from build123d import *

# Parameters (mm, degrees)
F0_W        = 5
F0_H        = 62.5
F0_H_2      = 5
F0_W_2      = 60
F1_DEPTH    = 10.5
F2_W        = 5
F2_H        = 62.5
F2_W_2      = 25
F2_W_3      = 65
F2_H_2      = 25
F3_DEPTH    = 4.75
F4_W        = 65
F4_H        = 25
F4_W_2      = 5
F4_H_2      = 62.5
F4_W_3      = 25
F5_DEPTH    = 4.75
F6_T1_DEPTH = 88.2168298797
F7_T1_DEPTH = 56.9578285833
F7_T3_DEPTH = 90.7168298797
F7_T5_DEPTH = 88.2168298797
F7_T7_DEPTH = 64.7680782592
F9_D        = 7


# Not quite as in the source:
# - a fillet or chamfer that OpenCascade refuses, or shapes differently, is made with other operations: its cross-section is extruded or revolved along the edge and cut away or added


with BuildPart() as f1:
    # F0 (on Top) → F1 (new body)
    with BuildSketch(Plane.XY):
        with Locations((0, 33.75)):
            Rectangle(F0_W, F0_H)
        Rectangle(F0_W, F0_H_2)
        with Locations((32.5, 0)):
            Rectangle(F0_W_2, F0_H_2)
    extrude(amount=F1_DEPTH)

    # F2 (on face) → F3 (join)
    with BuildSketch(Plane.XY.offset(10.5)):
        with Locations((0, 33.75)):
            Rectangle(F2_W, F2_H)
        Polygon((2.5, 2.5), (-2.5, 2.5), (-2.5, -2.5), (62.5, -2.5), (62.5, 2.5), align=None)
        Polygon((-2.5, -2.5), (-2.5, 2.5), (-27.5, 2.5), (-2.5, -27.5), align=None)
        with Locations((-15, 33.75)):
            Rectangle(F2_W_2, F2_H)
        with Locations((30, -15)):
            Rectangle(F2_W_3, F2_H_2)
    extrude(amount=F3_DEPTH)

    # F4 (on face) → F5 (join)
    with BuildSketch(Plane(origin=(0, 0, 0), x_dir=(1, 0, 0), z_dir=(0, 0, -1))):
        with Locations((30, 15)):
            Rectangle(F4_W, F4_H)
        Polygon((2.5, -2.5), (62.5, -2.5), (62.5, 2.5), (-2.5, 2.5), (-2.5, -2.5), align=None)
        Polygon((-27.5, -2.5), (-2.5, -2.5), (-2.5, 2.5), (-2.5, 27.5), align=None)
        with Locations((0, -33.75)):
            Rectangle(F4_W_2, F4_H_2)
        with Locations((-15, -33.75)):
            Rectangle(F4_W_3, F4_H_2)
    extrude(amount=F5_DEPTH)

    # F6: chamfer of 5 on 1 edges, made by hand

    # F6_s2 → F6_t1 (cut)
    with BuildSketch(Plane.XZ.offset(-77.8584149398)):
        Polygon((-27.5, 10.25), (-22.5, 15.25), (-27.5, 15.25), align=None)
    extrude(amount=F6_T1_DEPTH, mode=Mode.SUBTRACT)

    # F7: chamfer of 5 on 5 edges, made by hand

    # F7_s2 → F7_t1 (cut)
    with BuildSketch(Plane(origin=(-15.7317566489, 18.8781079787, 0), x_dir=(0, 0, 1), z_dir=(0.6401843997, -0.7682212796, 0))):
        Polygon((15.25, 14.5256241898), (10.25, 19.5256241898), (15.25, 19.5256241898), align=None)
    extrude(amount=F7_T1_DEPTH, mode=Mode.SUBTRACT)

    # F7_s4 → F7_t3 (cut)
    with BuildSketch(Plane.YZ.offset(-15.3584149398)):
        Polygon((-22.5, 15.25), (-27.5, 10.25), (-27.5, 15.25), align=None)
        Polygon((-22.5, -4.75), (-27.5, 0.25), (-27.5, -4.75), align=None)
    extrude(amount=F7_T3_DEPTH, mode=Mode.SUBTRACT)

    # F7_s6 → F7_t5 (cut)
    with BuildSketch(Plane.XZ.offset(-77.8584149398)):
        Polygon((-22.5, -4.75), (-27.5, 0.25), (-27.5, -4.75), align=None)
    extrude(amount=F7_T5_DEPTH, mode=Mode.SUBTRACT)

    # F7_s8 → F7_t7 (cut)
    with BuildSketch(Plane(origin=(20.7317566489, -24.8781079787, 0), x_dir=(0, 0, 1), z_dir=(-0.6401843997, 0.7682212796, 0))):
        Polygon((-4.75, -14.5256241898), (0.25, -19.5256241898), (-4.75, -19.5256241898), align=None)
    extrude(amount=F7_T7_DEPTH, mode=Mode.SUBTRACT)

    # F9 (through all)
    with Locations(Plane(origin=(0, 2.5, 0), x_dir=(-1, 0, 0), z_dir=(0, 1, 0))):
        with Locations((-14.02, 5.25)):
            Hole(F9_D / 2)


solid = f1.part
Design review of the part built by this model. Coordinates are the model's own, in mm. A direction names the side the tool comes from. Give positions to 0.01 mm unless a question says otherwise; leave off trailing zeros. Order: outer loops, then holes, each group sorted by start corner. A loop starts at its lowest first (then second) coordinate and runs counter-clockwise, first axis right, second up.
1. For pin 1 Ø1 at (y, z) = (6, 4) entering from +X; pin 2 Ø3 at (x, z) = (-3, 5.5) entering from -Y; pin 3 Ø1 at (y, z) = (21, 7.5) entering from -X, all flat-tipped, find the tip position at first contact; note any pin that passes through.
Solution:
pin 1: stops at x = 2.5
pin 2: stops at y = -2.5
pin 3: stops at x = -2.5
2. Mouldability with a two-part tool opening along Z and no side actions: class faces 1 (the flat face through (32, 2.5, 5)), 2 (the flat face through (-3, 8, 0)), 3 (the flat face through (-24.84, 34.23, -2.41)) as +Z half, -Z half, draft (parallel to the pull), parting line (faces both ways), or undercut.
Solution:
face 1: draft
face 2: undercut
face 3: -Z half
3. Tool access review of faces 4 (the flat face through (-2.5, 32, 5)), 5 (the flat face through (-3, 9, 10.5)), 6 (the flat face through (30, -2.5, 5)), 7 (the flat face through (2.5, 34, 5)): name each direction out of +Z, -Z, +X, -X, +Y, -Y from which nothing blocks a thin tool from reaching the whole face with its end or side.
Solution:
face 4: -X, +Y, -Y
face 5: -X, -Y
face 6: +X, -X, -Y
face 7: +Z, -Z, +X, +Y
4. Add section C-C, the plane y = 22. State the section outline as (x, z) points, then the cut area to 3 significant figures.
Solution:
outline: (-27.25, 0) - (-22.5, -4.75) - (2.5, -4.75) - (2.5, 15.25) - (-22.5, 15.25) - (-27.25, 10.5) - (-2.5, 10.5) - (-2.5, 0) - close
area: 313 mm2
5. Add section B-B, the plane x = 14.02. State the section outline as (y, z) points.
Solution:
outline: (-27.25, 0) - (-22.5, -4.75) - (2.5, -4.75) - (2.5, 1.75) - (-2.5, 1.75) - (-2.5, 0) - close; (-27.25, 10.5) - (-2.5, 10.5) - (-2.5, 8.75) - (2.5, 8.75) - (2.5, 15.25) - (-22.5, 15.25) - close
6. To check wall thickness, follow L1, parallel to Z at x = 26, y = -14.5; L2, parallel to Z at x = 14, y = 0; L3, parallel to X at y = 8.5, z = 7.5. State the ranges of each line that lie inside material, in increasing order.
Solution:
L1: z = -4.75 to 0, 10.5 to 15.25
L2: z = -4.75 to 1.75, 8.75 to 15.25
L3: x = -2.5 to 2.5
7. Add section A-A, the plane z = 5.25. State the section outline as (x, y) points, then the cut area to 4 significant figures.
Solution:
outline: (-2.5, -2.5) - (10.52, -2.5) - (10.52, 2.5) - (2.5, 2.5) - (2.5, 65) - (-2.5, 65) - close; (17.52, -2.5) - (62.5, -2.5) - (62.5, 2.5) - (17.52, 2.5) - close
area: 602.5 mm2
